from build123d import *

# Parameters (mm, degrees)
SKETCH1_R           = 1.7526
SKETCH1_W           = 9.525
SKETCH1_H           = 11.684
SKETCH1_W_2         = 6.35
SKETCH1_H_2         = 12.7
SKETCH1_W_3         = 5.741999946
SKETCH1_H_3         = 12.5
SKETCH1_W_4         = 5.842
SKETCH1_W_5         = 12.7
SKETCH1_H_4         = 5.842
BOSS_EXTRUDE1_DEPTH = 5.842
FILLET1_R           = 6.35
FILLET2_R           = 9.525
FILLET4_R           = 76.2
FILLET5_R           = 50.8
SKETCH2_W           = 9.525
SKETCH2_H           = 37.084
BOSS_EXTRUDE2_DEPTH = 5.842
SKETCH3_W           = 39.726031453
SKETCH3_H           = 13.117085857
BOSS_EXTRUDE3_DEPTH = 5.842
SKETCH4_W           = 12.5
SKETCH4_H           = 3.048
SKETCH4_W_2         = 3.048
SKETCH4_H_2         = 12.5
CUT_EXTRUDE1_DEPTH  = 158.941724336


with BuildPart() as part:
    # Sketch1 → Boss-Extrude1 (new body)
    with BuildSketch(Plane.XY):
        Polygon((25.4, 63.5), (-25.4, 63.5), (-25.4, 66.675), (-50.8, 73.9342438), (-139.446, 73.9342438), (-139.446, 16.7842438), (-127.254, 16.7842438), (-117.187573781, 36.3358938), (-70.673088246, 36.3358938), (-59.046135547, 13.75329052), (-44.45, -25.4), (44.45, -25.4), (59.046135547, 13.75329052), (70.673088246, 36.3358938), (117.187573781, 36.3358938), (127.254, 16.7842438), (139.446, 16.7842438), (139.446, 73.9342438), (50.8, 73.9342438), (25.4, 66.675), align=None)
        with Locations((28.370999973, 38.1)):
            Circle(SKETCH1_R, mode=Mode.SUBTRACT)
        with Locations(Location((-28.370999973, 38.1, 0), (0, 0, 180))):
            Circle(SKETCH1_R, mode=Mode.SUBTRACT)
        with Locations((-12.7, 41.275)):
            Circle(SKETCH1_R, mode=Mode.SUBTRACT)
        with Locations(Location((12.7, 41.275, 0), (0, 0, 180))):
            Circle(SKETCH1_R, mode=Mode.SUBTRACT)
        with Locations((-72.516999946, 50.7499874)):
            Circle(SKETCH1_R, mode=Mode.SUBTRACT)
        with Locations(Location((-40.766999946, 50.7499874, 0), (0, 0, 180))):
            Circle(SKETCH1_R, mode=Mode.SUBTRACT)
        with Locations((40.766999946, 50.7499874)):
            Circle(SKETCH1_R, mode=Mode.SUBTRACT)
        with Locations(Location((72.516999946, 50.7499874, 0), (0, 0, 180))):
            Circle(SKETCH1_R, mode=Mode.SUBTRACT)
        with Locations((133.35, 42.1842438)):
            Circle(SKETCH1_R, mode=Mode.SUBTRACT)
        with Locations(Location((-133.35, 42.1842438, 0), (0, 0, 180))):
            Circle(SKETCH1_R, mode=Mode.SUBTRACT)
        Polygon((25.5, -12.8), (18.95, -12.8), (18.95, -18.542), (6.45, -18.542), (6.45, -12.8), (-6.45, -12.8), (-6.45, -18.542), (-18.95, -18.542), (-18.95, -12.8), (-25.5, -12.8), (-25.5, -6.25), (-31.241999946, -6.25), (-31.241999946, 6.25), (-25.5, 6.25), (-25.5, 12.8), (-18.95, 12.8), (-18.95, 18.542), (-6.45, 18.542), (-6.45, 12.8), (6.45, 12.8), (6.45, 18.542), (18.95, 18.542), (18.95, 12.8), (25.5, 12.8), (25.5, 6.25), (31.241999946, 6.25), (31.241999946, -6.25), (25.5, -6.25), align=None, mode=Mode.SUBTRACT)
        with Locations((39.6875, 12.7)):
            Rectangle(SKETCH1_W, SKETCH1_H, mode=Mode.SUBTRACT)
        with Locations((39.6875, -12.7)):
            Rectangle(SKETCH1_W, SKETCH1_H, mode=Mode.SUBTRACT)
        with Locations((-39.6875, -12.7)):
            Rectangle(SKETCH1_W, SKETCH1_H, mode=Mode.SUBTRACT)
        with Locations((-39.6875, 12.7)):
            Rectangle(SKETCH1_W, SKETCH1_H, mode=Mode.SUBTRACT)
        with Locations((-12.7, 28.575)):
            Rectangle(SKETCH1_W_2, SKETCH1_H_2, mode=Mode.SUBTRACT)
        with Locations((-12.7, 53.975)):
            Rectangle(SKETCH1_W_2, SKETCH1_H_2, mode=Mode.SUBTRACT)
        with BuildLine():
            Line((82.55, 62.1930938), (92.075, 62.1930938))
            ThreePointArc((92.075, 62.1930938), (94.488, 59.7800938), (92.075, 57.3670938))
            Line((92.075, 57.3670938), (82.55, 57.3670938))
            ThreePointArc((82.55, 57.3670938), (80.137, 59.7800938), (82.55, 62.1930938))
        make_face(mode=Mode.SUBTRACT)
        with BuildLine():
            Line((82.55, 42.7620938), (92.075, 42.7620938))
            ThreePointArc((92.075, 42.7620938), (94.488, 40.3490938), (92.075, 37.9360938))
            Line((92.075, 37.9360938), (82.55, 37.9360938))
            ThreePointArc((82.55, 37.9360938), (80.137, 40.3490938), (82.55, 42.7620938))
        make_face(mode=Mode.SUBTRACT)
        with BuildLine():
            Line((107.95, 62.1930938), (117.475, 62.1930938))
            ThreePointArc((117.475, 62.1930938), (119.888, 59.7800938), (117.475, 57.3670938))
            Line((117.475, 57.3670938), (107.95, 57.3670938))
            ThreePointArc((107.95, 57.3670938), (105.537, 59.7800938), (107.95, 62.1930938))
        make_face(mode=Mode.SUBTRACT)
        with BuildLine():
            Line((107.95, 42.7620938), (117.475, 42.7620938))
            ThreePointArc((117.475, 42.7620938), (119.888, 40.3490938), (117.475, 37.9360938))
            Line((117.475, 37.9360938), (107.95, 37.9360938))
            ThreePointArc((107.95, 37.9360938), (105.537, 40.3490938), (107.95, 42.7620938))
        make_face(mode=Mode.SUBTRACT)
        Polygon((63.5, 73.1404938), (76.2, 73.1404938), (85.725, 73.1404938), (85.725, 69.9654938), (76.2, 69.9654938), (63.5, 69.9654938), align=None, mode=Mode.SUBTRACT)
        Polygon((114.3, 73.1404938), (127, 73.1404938), (136.525, 73.1404938), (136.525, 69.9654938), (127, 69.9654938), (114.3, 69.9654938), align=None, mode=Mode.SUBTRACT)
        with Locations((-28.370999973, 50.8)):
            Rectangle(SKETCH1_W_3, SKETCH1_H_3, mode=Mode.SUBTRACT)
        with Locations((-28.370999973, 25.4)):
            Rectangle(SKETCH1_W_3, SKETCH1_H_3, mode=Mode.SUBTRACT)
        with Locations((28.370999973, 50.8)):
            Rectangle(SKETCH1_W_3, SKETCH1_H_3, mode=Mode.SUBTRACT)
        with Locations((28.370999973, 25.4)):
            Rectangle(SKETCH1_W_3, SKETCH1_H_3, mode=Mode.SUBTRACT)
        with Locations((133.35, 29.4842438)):
            Rectangle(SKETCH1_W_4, SKETCH1_H_3, mode=Mode.SUBTRACT)
        with Locations((133.35, 54.8842438)):
            Rectangle(SKETCH1_W_4, SKETCH1_H_3, mode=Mode.SUBTRACT)
        Polygon((-127, 69.9654938), (-136.525, 69.9654938), (-136.525, 73.1404938), (-127, 73.1404938), (-114.3, 73.1404938), (-114.3, 69.9654938), align=None, mode=Mode.SUBTRACT)
        Polygon((-85.725, 73.1404938), (-85.725, 69.9654938), (-76.2, 69.9654938), (-63.5, 69.9654938), (-63.5, 73.1404938), (-76.2, 73.1404938), align=None, mode=Mode.SUBTRACT)
        with BuildLine():
            Line((-107.95, 42.7620938), (-117.475, 42.7620938))
            ThreePointArc((-117.475, 42.7620938), (-119.888, 40.3490938), (-117.475, 37.9360938))
            Line((-117.475, 37.9360938), (-107.95, 37.9360938))
            ThreePointArc((-107.95, 37.9360938), (-105.537, 40.3490938), (-107.95, 42.7620938))
        make_face(mode=Mode.SUBTRACT)
        with BuildLine():
            Line((-107.95, 62.1930938), (-117.475, 62.1930938))
            ThreePointArc((-117.475, 62.1930938), (-119.888, 59.7800938), (-117.475, 57.3670938))
            Line((-117.475, 57.3670938), (-107.95, 57.3670938))
            ThreePointArc((-107.95, 57.3670938), (-105.537, 59.7800938), (-107.95, 62.1930938))
        make_face(mode=Mode.SUBTRACT)
        with BuildLine():
            Line((-82.55, 42.7620938), (-92.075, 42.7620938))
            ThreePointArc((-92.075, 42.7620938), (-94.488, 40.3490938), (-92.075, 37.9360938))
            Line((-92.075, 37.9360938), (-82.55, 37.9360938))
            ThreePointArc((-82.55, 37.9360938), (-80.137, 40.3490938), (-82.55, 42.7620938))
        make_face(mode=Mode.SUBTRACT)
        with BuildLine():
            Line((-82.55, 62.1930938), (-92.075, 62.1930938))
            ThreePointArc((-92.075, 62.1930938), (-94.488, 59.7800938), (-92.075, 57.3670938))
            Line((-92.075, 57.3670938), (-82.55, 57.3670938))
            ThreePointArc((-82.55, 57.3670938), (-80.137, 59.7800938), (-82.55, 62.1930938))
        make_face(mode=Mode.SUBTRACT)
        with Locations((12.7, 28.575)):
            Rectangle(SKETCH1_W_2, SKETCH1_H_2, mode=Mode.SUBTRACT)
        with Locations((12.7, 53.975)):
            Rectangle(SKETCH1_W_2, SKETCH1_H_2, mode=Mode.SUBTRACT)
        with BuildLine():
            Line((-95.25, 69.8003938), (-104.775, 69.8003938))
            ThreePointArc((-104.775, 69.8003938), (-106.5276, 71.5529938), (-104.775, 73.3055938))
            Line((-104.775, 73.3055938), (-95.25, 73.3055938))
            ThreePointArc((-95.25, 73.3055938), (-93.4974, 71.5529938), (-95.25, 69.8003938))
        make_face(mode=Mode.SUBTRACT)
        with Locations((56.641999946, 50.7499874)):
            Rectangle(SKETCH1_W_5, SKETCH1_H_4, mode=Mode.SUBTRACT)
        with Locations((-56.641999946, 50.7499874)):
            Rectangle(SKETCH1_W_5, SKETCH1_H_4, mode=Mode.SUBTRACT)
        with BuildLine():
            Line((95.25, 69.8003938), (104.775, 69.8003938))
            ThreePointArc((104.775, 69.8003938), (106.5276, 71.5529938), (104.775, 73.3055938))
            Line((104.775, 73.3055938), (95.25, 73.3055938))
            ThreePointArc((95.25, 73.3055938), (93.4974, 71.5529938), (95.25, 69.8003938))
        make_face(mode=Mode.SUBTRACT)
        with Locations((-133.35, 29.4842438)):
            Rectangle(SKETCH1_W_4, SKETCH1_H_3, mode=Mode.SUBTRACT)
        with Locations((-133.35, 54.8842438)):
            Rectangle(SKETCH1_W_4, SKETCH1_H_3, mode=Mode.SUBTRACT)
    extrude(amount=BOSS_EXTRUDE1_DEPTH)

    # Fillet1
    fillet1_edges = [part.edges().sort_by_distance(p)[0] for p in [
        (70.673088246, 36.3358938, 2.921),
        (-70.673088246, 36.3358938, 2.921),
    ]]
    fillet(fillet1_edges, radius=FILLET1_R)

    # Fillet2
    fillet2_edges = [part.edges().sort_by_distance(p)[0] for p in [
        (44.45, -25.4, 2.921),
        (-44.45, -25.4, 2.921),
    ]]
    fillet(fillet2_edges, radius=FILLET2_R)

    # Fillet4
    fillet4_edges = [part.edges().sort_by_distance(p)[0] for p in [
        (50.8, 73.9342438, 2.921),
        (-50.8, 73.9342438, 2.921),
    ]]
    fillet(fillet4_edges, radius=FILLET4_R)

    # Fillet5
    fillet5_edges = [part.edges().sort_by_distance(p)[0] for p in [
        (59.046135547, 13.75329052, 2.921),
        (-59.046135547, 13.75329052, 2.921),
    ]]
    fillet(fillet5_edges, radius=FILLET5_R)

    # Sketch2 → Boss-Extrude2 (add)
    with BuildSketch(Plane.XY.offset(5.842)):
        with Locations((-39.6875, 0)):
            Rectangle(SKETCH2_W, SKETCH2_H)
        with Locations((39.6875, 0)):
            Rectangle(SKETCH2_W, SKETCH2_H)
    extrude(amount=-BOSS_EXTRUDE2_DEPTH)

    # Sketch3 → Boss-Extrude3 (add)
    with BuildSketch(Plane.XY.offset(5.842)):
        with Locations((-57.1552409, 51.348468537)):
            Rectangle(SKETCH3_W, SKETCH3_H)
        Polygon((-31.241999946, 57.05), (-25.5, 57.05), (-25.5, 19.15), (-25.5, -6.25), (-31.241999946, -6.25), (-31.241999946, 19.15), align=None)
        Polygon((25.5, 57.05), (25.5, 19.15), (25.5, -6.25), (31.241999946, -6.25), (31.241999946, 19.15), (31.241999946, 57.05), align=None)
        with Locations((57.1552409, 51.348468537)):
            Rectangle(SKETCH3_W, SKETCH3_H)
    extrude(amount=-BOSS_EXTRUDE3_DEPTH)

    # Sketch4 → Cut-Extrude1 (cut, through all)
    with BuildSketch(Plane.XY.offset(5.842)):
        with Locations((44.45, 61.976)):
            Rectangle(SKETCH4_W, SKETCH4_H)
        with Locations((-44.45, 61.976)):
            Rectangle(SKETCH4_W, SKETCH4_H)
        with Locations((-25.4, 49.276)):
            Rectangle(SKETCH4_W_2, SKETCH4_H_2)
        with Locations((25.4, 49.276)):
            Rectangle(SKETCH4_W_2, SKETCH4_H_2)
    extrude(amount=-CUT_EXTRUDE1_DEPTH, mode=Mode.SUBTRACT)


solid = part.part
Source: CAD feature listing. Evaluate the final solid. Frame: model axes, mm. A direction names the side the tool comes from. Coordinates: 2 decimals unless noted, no trailing zeros. Loops run counter-clockwise (first coordinate to the right, second up) from the corner with the lowest first, then second, coordinate; pieces in that order, holes last. Notation, with made-up numbers: (70, -3) -> (88, -3) arc R16 ccw to (88, 4) -> close; hole circle Ø2 at (46, 7.25). An arc over 180 degrees is marked (long way). Answer in a Markdown table with one row per item. Add a question column.
Q1. Reachability of faces 4 (the face through (-71.28, 35.43, 2.96)), 5 (the face through (23.876, 49, 3)) from +Z, -Z, +X, -X, +Y, -Y: full face, straight path, thin tool, end or side. Return the list, or none.
Q2. Section B-B on x = 111.5. Return the cut outline in (y, z).
Q3. Pull-direction query (X, two-part tool) for faces 1 (the face through (101, 73.934, 3)), 2 (the face through (-130.429, 29, 3)), 3 (the face through (139.446, 45, 3)); classes: pulls with the +X half, pulls with the -X half, needs draft (parallel to the pull), parting line crosses it, or undercut.
Q4. Ray query, line 1 along Y through (x, z) = (-12.7, 1.65) (3 decimals); line 2 along Y through (x, z) = (133.35, 4.6); line 3 along X through (y, z) = (56, 3.95) (3 decimals). Return the intervals inside material, ascending.
Q5. Section A-A on x = -1. Return the cut outline in (y, z), and give its area (3 significant figures).
Q6. Section D-D on y = 28.5. Return the cut outline in (x, z) (3 decimals).
Q7. Contact query for flat-ended pins moving along their axis: pin 1 Ø1.7 at (y, z) = (16, 3) entering from +X; pin 2 Ø1.8 at (x, z) = (100, 3) entering from -Y. Output: stop coordinate, or through.
Q8. Section C-C on y = -3.5. Return the cut outline in (x, z), and give its area (3 significant figures).
Computed values:
| question | item | result |
|---|---|---|
| 1 | face 4 | +Z, -Z, -Y |
| 1 | face 5 | +Z, -Z |
| 2 | outline | (36.34, 0) -> (37.94, 0) -> (37.94, 5.84) -> (36.34, 5.84) -> close; (42.76, 0) -> (57.37, 0) -> (57.37, 5.84) -> (42.76, 5.84) -> close; (62.19, 0) -> (73.93, 0) -> (73.93, 5.84) -> (62.19, 5.84) -> close |
| 3 | face 1 | needs draft |
| 3 | face 2 | undercut |
| 3 | face 3 | pulls with the +X half |
| 4 | line 1 | y = -25.4 to -18.542, 18.542 to 22.225, 34.925 to 39.522, 43.028 to 47.625, 60.325 to 63.5 |
| 4 | line 2 | y = 16.78 to 23.23, 35.73 to 40.43, 43.94 to 48.63, 61.13 to 69.97, 73.14 to 73.93 |
| 4 | line 3 | x = -139.446 to -136.271, -130.429 to -15.875, -9.525 to 9.525, 15.875 to 130.429, 136.271 to 139.446 |
| 5 | outline | (-25.4, 0) -> (-12.8, 0) -> (-12.8, 5.84) -> (-25.4, 5.84) -> close; (12.8, 0) -> (63.5, 0) -> (63.5, 5.84) -> (12.8, 5.84) -> close |
| 5 | area | 370 mm^2 |
| 6 | outline | (-139.446, 0) -> (-136.271, 0) -> (-136.271, 5.842) -> (-139.446, 5.842) -> close; (-130.429, 0) -> (-121.222, 0) -> (-121.222, 5.842) -> (-130.429, 5.842) -> close; (-66.639, 0) -> (-15.875, 0) -> (-15.875, 5.842) -> (-66.639, 5.842) -> close; (-9.525, 0) -> (9.525, 0) -> (9.525, 5.842) -> (-9.525, 5.842) -> close; (15.875, 0) -> (66.639, 0) -> (66.639, 5.842) -> (15.875, 5.842) -> close; (121.222, 0) -> (130.429, 0) -> (130.429, 5.842) -> (121.222, 5.842) -> close; (136.271, 0) -> (139.446, 0) -> (139.446, 5.842) -> (136.271, 5.842) -> close |
| 7 | pin 1 | stops at x = 139.45 |
| 7 | pin 2 | stops at y = 36.34 |
| 8 | outline | (-52.61, 0) -> (-25.5, 0) -> (-25.5, 5.84) -> (-52.61, 5.84) -> close; (25.5, 0) -> (52.61, 0) -> (52.61, 5.84) -> (25.5, 5.84) -> close |
| 8 | area | 317 mm^2 |
